Build history of the part. All positions in model axes, mm. A direction names the side the tool comes from. Round coordinates to 2 decimals unless told otherwise and drop trailing zeros. Write each loop counter-clockwise with the first axis right and the second up, starting at its lowest first coordinate (ties: lowest second). Pieces come first, ordered by that corner, then holes. Notation, with made-up numbers: M -29,53.25 L -14,53.25 A15 ccw -14,79.25 Z; hole C -15.75,-23 d10. An arc over 180 degrees is marked long. One line per item, written item: value. Start each with the question number.
```python
from build123d import *

# Parameters (mm, degrees)
CROQUIS1_R              = 75
SALIENTE_EXTRUIR1_DEPTH = 40
SALIENTE_EXTRUIR2_START = 5
CROQUIS3_R              = 46.15
SALIENTE_EXTRUIR2_DEPTH = 36.5
CROQUIS5_R              = 51
CROQUIS5_R_2            = 41
SALIENTE_EXTRUIR3_DEPTH = 10
CHAFL_N1_SIZE           = 5.350722602
CHAFL_N1_SIZE_2         = 10
CHAFL_N2_SIZE2          = 10
CHAFL_N2_SIZE           = 5.350722602
REDONDEO1_R             = 5
CROQUIS7_R              = 2.248271999
CROQUIS7_R_2            = 2.28310755
CORTAR_EXTRUIR2_DEPTH   = 212.91154603
CROQUIS8_R              = 61.227064255
CORTAR_EXTRUIR3_DEPTH   = 1.5
CROQUIS8_3_R            = 2.5
CORTAR_EXTRUIR4_DEPTH   = 10


# Some blends are built 0.0001 mm under size
with BuildPart() as part:
    # Croquis1 → Saliente-Extruir1 (new body)
    with BuildSketch(Plane(origin=(0, 0, 0), x_dir=(1, 0, 0), z_dir=(0, 1, 0))):
        with Locations(Location((0, 0, 0), (0, 0, 270))):
            Circle(CROQUIS1_R)
    extrude(amount=SALIENTE_EXTRUIR1_DEPTH)

    # Croquis3 → Saliente-Extruir2 (add)
    with BuildSketch(Plane.XY.offset(SALIENTE_EXTRUIR2_START)):
        with BuildLine():
            Line((45, 146.000391386), (43.906975528, 146.000391386))
            ThreePointArc((43.906975528, 146.000391386), (0, 167.150391386), (-43.906975528, 146.000391386))
            Line((-43.906975528, 146.000391386), (-45, 146.000391386))
            ThreePointArc((-45, 146.000391386), (-48.535533906, 144.535925292), (-50, 141.000391386))
            Line((-50, 141.000391386), (-50, 136.550782773))
            ThreePointArc((-50, 136.550782773), (-56.15, 111.000391386), (-50, 85.45))
            Line((-50, 85.45), (-50, 40))
            Line((-50, 40), (50, 40))
            Line((50, 40), (50, 85.45))
            ThreePointArc((50, 85.45), (56.15, 111.000391386), (50, 136.550782773))
            Line((50, 136.550782773), (50, 141.000391386))
            ThreePointArc((50, 141.000391386), (48.535533906, 144.535925292), (45, 146.000391386))
        make_face()
        with Locations((0, 111.000391386)):
            Circle(CROQUIS3_R, mode=Mode.SUBTRACT)
    extrude(amount=-SALIENTE_EXTRUIR2_DEPTH)

    # Croquis5 → Saliente-Extruir3 (add)
    with BuildSketch(Plane.XY.offset(5)):
        with Locations((0, 111.000391386)):
            Circle(CROQUIS5_R)
        with Locations((0, 111.000391386)):
            Circle(CROQUIS5_R_2, mode=Mode.SUBTRACT)
    extrude(amount=SALIENTE_EXTRUIR3_DEPTH)

    # Chaflán1
    # the kernel refuses this chamfer: 10, 5.350722602 mm, written as the material it takes off along each edge
    with BuildSketch(Plane(origin=(0, 111.000391386, 5), x_dir=(1, 0, 0), z_dir=(0, -1, 0))) as chafl_n1_piece_1_section:
        Polygon((41 + CHAFL_N1_SIZE, 0), (41, CHAFL_N1_SIZE_2), (41, 0), align=None)
    chafl_n1_piece_1 = revolve(axis=Axis((0, 111.000391386, 5), (0, 0, 1)), mode=Mode.PRIVATE)
    chafl_n1_piece_1 = chafl_n1_piece_1 & Plane(origin=(0, 111.000391386, 10.096546519), x_dir=(1, 0, 0), z_dir=(0, 0, 1)) * Cylinder(46.15, 186, mode=Mode.PRIVATE)
    add(chafl_n1_piece_1, mode=Mode.SUBTRACT)

    # Chaflán2
    chafl_n2_edges = [part.edges().sort_by_distance(p)[0] for p in [
        (-51, 111.000391386, 15),
    ]]
    chafl_n2_side = [part.faces().sort_by_distance(p)[0] for p in [
        (-50.892985548, 111.000391386, 15),
    ]]
    chamfer(chafl_n2_edges, length=CHAFL_N2_SIZE - 0.0001, length2=CHAFL_N2_SIZE2 - 0.0001, reference=chafl_n2_side[0])  # a hair under: the kernel refuses the full size

    # Redondeo1
    redondeo1_edges = [part.edges().sort_by_distance(p)[0] for p in [
        (0, 40, 5),
        (0, 40, -31.5),
        (50, 40, -13.25),
        (-50, 40, -13.25),
    ]]
    fillet(redondeo1_edges, radius=REDONDEO1_R)

    # Croquis7 → Cortar-Extruir2 (cut, through all)
    with BuildSketch(Plane(origin=(0, 0, -31.5), x_dir=(-1, 0, 0), z_dir=(0, 0, -1))):
        with Locations((45, 141.000391386)):
            Circle(CROQUIS7_R)
        with Locations((-45.000000475, 141.000390201)):
            Circle(CROQUIS7_R_2)
        with Locations(Location((-45.000000475, 80.973259529, 0), (0, 0, 180))):
            Circle(CROQUIS7_R_2)
        with Locations(Location((45, 80.973258343, 0), (0, 0, 180))):
            Circle(CROQUIS7_R)
    extrude(amount=-CORTAR_EXTRUIR2_DEPTH, mode=Mode.SUBTRACT)

    # Croquis8 → Cortar-Extruir3 (cut)
    with BuildSketch(Plane.XZ):
        with Locations(Location((0, 0, 0), (0, 0, 270))):
            Circle(CROQUIS8_R)
    extrude(amount=-CORTAR_EXTRUIR3_DEPTH, mode=Mode.SUBTRACT)

    # Croquis8<3> → Cortar-Extruir4 (cut)
    with BuildSketch(Plane.XZ):
        with Locations(Location((-2.647399238, 28.274392606, 0), (0, 0, 270))):
            Circle(CROQUIS8_3_R)
        with Locations(Location((24.207953628, -14.846716173, 0), (0, 0, 270))):
            Circle(CROQUIS8_3_R)
        with Locations(Location((2.647399238, -28.274392607, 0), (0, 0, 270))):
            Circle(CROQUIS8_3_R)
        with Locations(Location((-24.207953628, 14.846716173, 0), (0, 0, 270))):
            Circle(CROQUIS8_3_R)
    extrude(amount=-CORTAR_EXTRUIR4_DEPTH, mode=Mode.SUBTRACT)


solid = part.part
```
Item 1: Cut at B-B, the plane z = -55.5. Write the cut outline in (x, y).
Item 2: Drill centre lines: line 1 (Y direction, x = 0, z = -12.5); line 2 (Y direction, x = 2, z = -13); line 3 (Z direction, x = 26.5, y = 156). Where is each one in solid material? Low to high.
Item 3: Drop flat-ended pins along their axis: pin 1 (6 mm diameter, centred on x = -45, y = 80.97, fed in from +Z); pin 2 (4 mm diameter, centred on x = -35, z = -24.5, fed in from +Y); pin 3 (1.5 mm diameter, centred on x = -24.5, z = 14, fed in from -Y); pin 4 (6.5 mm diameter, centred on x = 2.65, z = -28.27, fed in from +Y). Give the stop position or say it passes through.
Item 4: Cut at A-A, the plane z = 0. Write the cut outline in (x, y).
Item 5: Cut at D-D, the plane z = 34.5. Write the cut outline in (x, y).
Item 6: Two-plate mould, pull along Z, no slides. Class faces 1 (the flat face through (12, 66, -31.5)), 2 (the cylindrical face through (51, 42, -14)), 3 (the flat face through (-24, 10, 15)), 4 (the cylindrical face through (-2.537, 5.69, 30.772)): pulls with the +Z half, pulls with the -Z half, needs draft (parallel to the pull), parting line crosses it, or undercut.
Item 7: Which spindle directions (+Z, -Z, +X, -X, +Y, -Y) get a long thin tool onto all of the face, cutting with end or side? Do faces 5 (the flat face through (-50, 139, -13)), 6 (the flat face through (-3, 10, 28)), 7 (the flat face through (12, 61, 5)), 8 (the cylindrical face through (-52, 41, -14)), 9 (the flat face through (50, 139, -13)). Say none if no direction does.
Item 8: Cut at C-C, the plane y = 30.5. Write the cut outline in (x, z), plus the area to 3 significant figures.
Computed values:
1. outline: M -50.45,0 L -25.86,0 L -25.86,1.5 L 25.86,1.5 L 25.86,0 L 50.45,0 L 50.45,40 L -50.45,40 Z
2. line 1: y = 1.5 to 64.85, 157.15 to 167.15
2. line 2: y = 1.5 to 64.89, 157.11 to 167.11
2. line 3: z = -31.5 to 5
3. pin 1: stops at z = 5
3. pin 2: stops at y = 156.43
3. pin 3: stops at y = 10
3. pin 4: stops at y = 167.15
4. outline: M -75,0 L -61.23,0 L -61.23,1.5 L 61.23,1.5 L 61.23,0 L 75,0 L 75,40 L 55,40 A5 cw 50,45 L 50,85.45 A56.15 ccw 50,136.55 L 50,141 A5 ccw 45,146 L 43.91,146 A56.15 ccw -43.91,146 L -45,146 A5 ccw -50,141 L -50,136.55 A56.15 ccw -50,85.45 L -50,45 A5 cw -55,40 L -75,40 Z; hole C -45,80.97 d4.5; hole C -45,141 d4.5; hole C 0,111 d92.3; hole C 45,80.97 d4.57; hole C 45,141 d4.57
5. outline: M -66.59,0 L -50.58,0 L -50.58,1.5 L 50.58,1.5 L 50.58,0 L 66.59,0 L 66.59,40 L -66.59,40 Z
6. face 1: pulls with the -Z half
6. face 2: needs draft
6. face 3: undercut
6. face 4: undercut
7. face 5: +Z, -Z, -X, +Y
7. face 6: -Y
7. face 7: +Z
7. face 8: +Z, -Z, -X
7. face 9: +Z, -Z, +X, +Y
8. outline: C 0,0 d150
8. area: 17,700 mm2
